The model under review builds one solid part; all positions refer to its coordinate system, in mm. Face numbers are marked on the shaded views. Coordinates: 2 decimals unless noted, no trailing zeros. Loops run counter-clockwise (first coordinate to the right, second up) from the corner with the lowest first, then second, coordinate; pieces in that order, holes last. Notation, with made-up numbers: M 26,82 L 57,82 A16 ccw 57,100 Z; hole C -35.5,-3 d11. An arc over 180 degrees is marked long. Use one line per item in the form item = value.
```python
from build123d import *

# Parameters (mm, degrees)
F0_W     = 177.8
F0_H     = 114.3
F1_DEPTH = 6.35
F2_R     = 3.17499
F3_T     = -2.54


# Not quite as in the source:
# - a fillet or chamfer is up to 0.001 mm smaller than in the source, because OpenCascade refuses the exact size
# - a shell that OpenCascade refuses in one call is made with other operations: the cavity is built on its own and cut out


with BuildPart() as f1:
    # F0 (on Front) → F1 (new body)
    with BuildSketch(Plane.XZ):
        with Locations((45.9769070864, 28.9183518412)):
            Rectangle(F0_W, F0_H)
    extrude(amount=F1_DEPTH)

    # F2 (radius 3.175 in the source; OpenCascade refuses exactly that, so slightly less here)
    f2_edges = [f1.edges().sort_by_distance(p)[0] for p in [
        (45.976907, 0, 86.068352),
        (134.876907, -3.175, 86.068352),
        (45.976907, -6.35, 86.068352),
        (-42.923093, -3.175, 86.068352),
        (-42.923093, -6.35, 28.918352),
        (134.876907, -6.35, 28.918352),
        (134.876907, 0, 28.918352),
        (45.976907, -6.35, -28.231648),
        (45.976907, 0, -28.231648),
        (-42.923093, 0, 28.918352),
        (134.876907, -3.175, -28.231648),
        (-42.923093, -3.175, -28.231648),
    ]]
    fillet(f2_edges, radius=F2_R)

    # F3: a shell. OpenCascade refuses it in one call, so the cavity is built on its own and cut out:
    # the body offset inwards by the wall thickness, plus a prism from it out through each open face.
    f3_core = offset(f1.part, amount=F3_T, mode=Mode.PRIVATE)
    f3_exits = [f3_core.faces().sort_by_distance(p)[0] for p in [
        (45.976907, -3.81, 28.918352),
    ]]
    add(f3_core, mode=Mode.SUBTRACT)
    extrude(f3_exits, amount=-F3_T, mode=Mode.SUBTRACT)


solid = f1.part
```
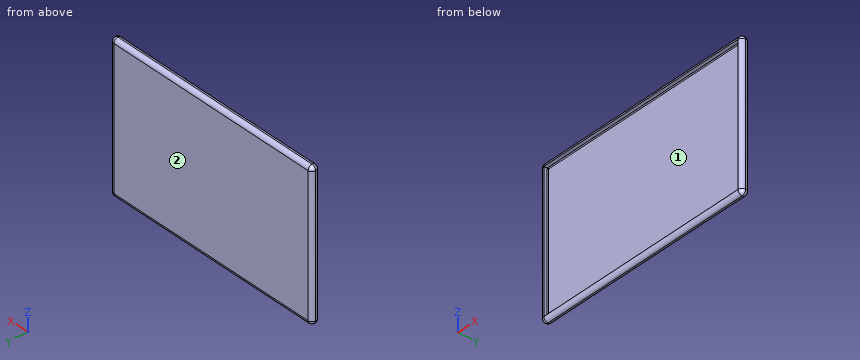
1. The part is to be moulded in two halves that separate along X. For the marked faces 1 and 2, say which applies: pulls with the +X half, pulls with the -X half, needs draft (parallel to the pull), parting line crosses it, or undercut.
Response values:
face_1 = undercut
face_2 = needs draft
2. Add section C-C (y = -5). State the section outline as (x, z) points, then the cut area to 3 significant figures.
Response values:
outline = M -42.35,-25.06 A2.6 ccw -39.75,-27.65 L 131.7,-27.65 A2.6 ccw 134.3,-25.06 L 134.3,82.89 A2.6 ccw 131.7,85.49 L -39.75,85.49 A2.6 ccw -42.35,82.89 Z; hole M -39.75,-25.06 L 131.7,-25.06 L 131.7,82.89 L -39.75,82.89 Z
area = 1,470 mm^2
3. Wall thickness on line 1 along Y through (x, z) = (-28, 77.5); line 2 along X through (y, z) = (-2.75, 32); line 3 along Z through (x, y) = (58, -3.5): over which ranges is each line inside the solid? List them lowest first. Write a range as from..to.
Response values:
line_1 = -2.54..0
line_2 = -42.89..-40.22, 132.17..134.85
line_3 = -28.21..-25.6, 83.44..86.05
4. Insertion check: P1, Ø3, axis at y = -5.5, z = 14, coming from the -X side; P2, Ø2, axis at y = -2, z = 65, coming from the +X side; P3, Ø3, axis at y = -2, z = -4, coming from the -X side; P4, Ø2, axis at x = 57.5, y = -5, coming from the +Z side. Each pin has a flat end and moves straight along its axis. Give the tip position at first contact, or say it passes through.
Response values:
P1 = -42.81
P2 = 134.87
P3 = -42.92
P4 = 85.96
